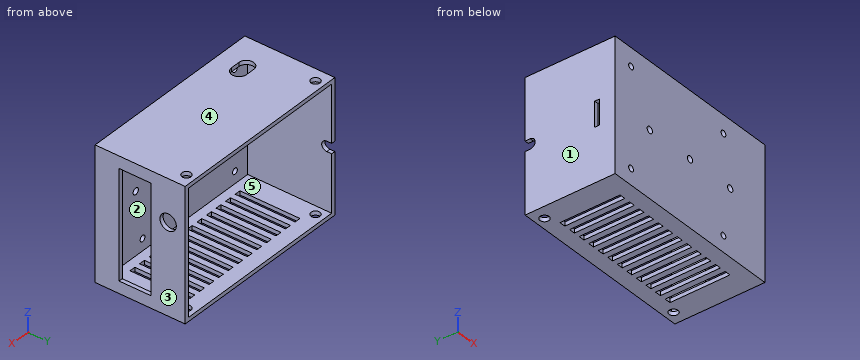
from build123d import *

# Parameters (mm, degrees)
SKETCH1_W           = 90
SKETCH1_H           = 62
BOSS_EXTRUDE1_DEPTH = 3
CUT_EXTRUDE1_REACH  = 56.727
SKETCH2_R           = 1.5
SKETCH3_W           = 94
SKETCH3_H           = 66
SKETCH3_W_2         = 90
SKETCH3_H_2         = 62
BOSS_EXTRUDE2_DEPTH = 45
CUT_EXTRUDE2_REACH  = 109.601
SKETCH4_W           = 12.5
SKETCH4_H           = 2.5
CUT_EXTRUDE3_REACH  = 93.269
CUT_EXTRUDE4_REACH  = 109.601
SKETCH6_W           = 54
SKETCH6_H           = 16
CUT_EXTRUDE5_REACH  = 111.316
SKETCH7_R           = 4.1
SKETCH8_R           = 2.25
CUT_EXTRUDE6_DEPTH  = 93.682252886
CUT_EXTRUDE7_DEPTH  = 72.147733625
CUT_EXTRUDE8_REACH  = 94.682
SKETCH10_W          = 3
SKETCH10_H          = 30
CUT_EXTRUDE9_REACH  = 111.316


with BuildPart() as part:
    # Sketch1 → Boss-Extrude1 (new body)
    with BuildSketch(Plane(origin=(0, 0, 0), x_dir=(1, 0, 0), z_dir=(0, 1, 0))):
        Rectangle(SKETCH1_W, SKETCH1_H)
    extrude(amount=BOSS_EXTRUDE1_DEPTH)

    # Sketch2 → Cut-Extrude1 (cut, up to next)
    with BuildSketch(Plane(origin=(0, 3, 0), x_dir=(1, 0, 0), z_dir=(0, 1, 0)), mode=Mode.PRIVATE) as cut_extrude1_sk1:
        with Locations(Location((-37, -24, 0), (0, 0, 270))):
            Circle(SKETCH2_R)
    cut_extrude1_tool1 = extrude(cut_extrude1_sk1.sketch, amount=-CUT_EXTRUDE1_REACH, mode=Mode.PRIVATE) & part.part
    # Sketch2 → Cut-Extrude1 (cut, up to next)
    with BuildSketch(Plane(origin=(0, 3, 0), x_dir=(1, 0, 0), z_dir=(0, 1, 0)), mode=Mode.PRIVATE) as cut_extrude1_sk2:
        with Locations(Location((21, -24, 0), (0, 0, 270))):
            Circle(SKETCH2_R)
    cut_extrude1_tool2 = extrude(cut_extrude1_sk2.sketch, amount=-CUT_EXTRUDE1_REACH, mode=Mode.PRIVATE) & part.part
    # Sketch2 → Cut-Extrude1 (cut, up to next)
    with BuildSketch(Plane(origin=(0, 3, 0), x_dir=(1, 0, 0), z_dir=(0, 1, 0)), mode=Mode.PRIVATE) as cut_extrude1_sk3:
        with Locations(Location((21, 25, 0), (0, 0, 270))):
            Circle(SKETCH2_R)
    cut_extrude1_tool3 = extrude(cut_extrude1_sk3.sketch, amount=-CUT_EXTRUDE1_REACH, mode=Mode.PRIVATE) & part.part
    # Sketch2 → Cut-Extrude1 (cut, up to next)
    with BuildSketch(Plane(origin=(0, 3, 0), x_dir=(1, 0, 0), z_dir=(0, 1, 0)), mode=Mode.PRIVATE) as cut_extrude1_sk4:
        with Locations(Location((-37, 25, 0), (0, 0, 270))):
            Circle(SKETCH2_R)
    cut_extrude1_tool4 = extrude(cut_extrude1_sk4.sketch, amount=-CUT_EXTRUDE1_REACH, mode=Mode.PRIVATE) & part.part
    add(cut_extrude1_tool1.solids().sort_by_distance((-37, 3, 24))[0], mode=Mode.SUBTRACT)
    add(cut_extrude1_tool2.solids().sort_by_distance((21, 3, 24))[0], mode=Mode.SUBTRACT)
    add(cut_extrude1_tool3.solids().sort_by_distance((21, 3, -25))[0], mode=Mode.SUBTRACT)
    add(cut_extrude1_tool4.solids().sort_by_distance((-37, 3, -25))[0], mode=Mode.SUBTRACT)

    # Sketch3 → Boss-Extrude2 (add)
    with BuildSketch(Plane(origin=(0, 0, 0), x_dir=(1, 0, 0), z_dir=(0, 1, 0))):
        Rectangle(SKETCH3_W, SKETCH3_H)
        Rectangle(SKETCH3_W_2, SKETCH3_H_2, mode=Mode.SUBTRACT)
    extrude(amount=BOSS_EXTRUDE2_DEPTH)

    # Sketch4 → Cut-Extrude2 (cut, up to next)
    with BuildSketch(Plane(origin=(-45, 0, 0), x_dir=(0, 0, -1), z_dir=(1, 0, 0)), mode=Mode.PRIVATE) as cut_extrude2_sk1:
        with Locations((0, 9)):
            Rectangle(SKETCH4_W, SKETCH4_H)
    cut_extrude2_tool1 = extrude(cut_extrude2_sk1.sketch, amount=-CUT_EXTRUDE2_REACH, mode=Mode.PRIVATE) & part.part
    add(cut_extrude2_tool1.solids().sort_by_distance((-45, 9, 0))[0], mode=Mode.SUBTRACT)

    # Sketch5 → Cut-Extrude3 (cut, up to next)
    with BuildSketch(Plane(origin=(0, 0, 31), x_dir=(-1, 0, 0), z_dir=(0, 0, -1)), mode=Mode.PRIVATE) as cut_extrude3_sk1:
        with BuildLine():
            Line((31.55, 9.25), (27.05, 9.25))
            ThreePointArc((27.05, 9.25), (23.3, 13), (27.05, 16.75))
            Line((27.05, 16.75), (31.55, 16.75))
            ThreePointArc((31.55, 16.75), (35.3, 13), (31.55, 9.25))
        make_face()
    cut_extrude3_tool1 = extrude(cut_extrude3_sk1.sketch, amount=-CUT_EXTRUDE3_REACH, mode=Mode.PRIVATE) & part.part
    add(cut_extrude3_tool1.solids().sort_by_distance((-29.3, 13, 31))[0], mode=Mode.SUBTRACT)

    # Sketch6 → Cut-Extrude4 (cut, up to next)
    with BuildSketch(Plane.ZY.offset(-45), mode=Mode.PRIVATE) as cut_extrude4_sk1:
        with Locations((0, 20)):
            Rectangle(SKETCH6_W, SKETCH6_H)
    cut_extrude4_tool1 = extrude(cut_extrude4_sk1.sketch, amount=-CUT_EXTRUDE4_REACH, mode=Mode.PRIVATE) & part.part
    add(cut_extrude4_tool1.solids().sort_by_distance((45, 20, 0))[0], mode=Mode.SUBTRACT)

    # Sketch7 → Cut-Extrude5 (cut, up to next)
    with BuildSketch(Plane(origin=(47, 0, 0), x_dir=(0, 0, -1), z_dir=(1, 0, 0)), mode=Mode.PRIVATE) as cut_extrude5_sk1:
        with Locations((-12, 36.5)):
            Circle(SKETCH7_R)
    cut_extrude5_tool1 = extrude(cut_extrude5_sk1.sketch, amount=-CUT_EXTRUDE5_REACH, mode=Mode.PRIVATE) & part.part
    add(cut_extrude5_tool1.solids().sort_by_distance((47, 36.5, 12))[0], mode=Mode.SUBTRACT)

    # Sketch8 → Cut-Extrude6 (cut, through all)
    with BuildSketch(Plane.XY.offset(33)):
        with Locations((-40.5, 40.5)):
            Circle(SKETCH8_R)
        with Locations(Location((40.5, 40.5, 0), (0, 0, 180))):
            Circle(SKETCH8_R)
    extrude(amount=-CUT_EXTRUDE6_DEPTH, mode=Mode.SUBTRACT)

    # Sketch9 → Cut-Extrude7 (cut, through all)
    with BuildSketch(Plane(origin=(0, 3, 0), x_dir=(1, 0, 0), z_dir=(0, 1, 0))):
        with BuildLine():
            ThreePointArc((-23.6, 0), (-25.25, 1.65), (-26.9, 0))
            Line((-26.9, 0), (-23.6, 0))
        make_face()
        with BuildLine():
            Line((-23.6, 0), (-26.9, 0))
            ThreePointArc((-26.9, 0), (-25.25, -1.65), (-23.6, 0))
        make_face()
        with BuildLine():
            ThreePointArc((1.65, 0), (0, 1.65), (-1.65, 0))
            Line((-1.65, 0), (1.65, 0))
        make_face()
        with BuildLine():
            Line((1.65, 0), (-1.65, 0))
            ThreePointArc((-1.65, 0), (0, -1.65), (1.65, 0))
        make_face()
        with BuildLine():
            ThreePointArc((26.9, 0), (25.25, 1.65), (23.6, 0))
            Line((23.6, 0), (26.9, 0))
        make_face()
        with BuildLine():
            Line((26.9, 0), (23.6, 0))
            ThreePointArc((23.6, 0), (25.25, -1.65), (26.9, 0))
        make_face()
    extrude(amount=-CUT_EXTRUDE7_DEPTH, mode=Mode.SUBTRACT)

    # Sketch10 → Cut-Extrude8 (cut, up to next)
    with BuildSketch(Plane(origin=(0, 0, -33), x_dir=(-1, 0, 0), z_dir=(0, 0, -1)), mode=Mode.PRIVATE) as cut_extrude8_sk1:
        with Locations((9, 22.5)):
            Rectangle(SKETCH10_W, SKETCH10_H)
    cut_extrude8_tool1 = extrude(cut_extrude8_sk1.sketch, amount=-CUT_EXTRUDE8_REACH, mode=Mode.PRIVATE) & part.part
    # Sketch10 → Cut-Extrude8 (cut, up to next)
    with BuildSketch(Plane(origin=(0, 0, -33), x_dir=(-1, 0, 0), z_dir=(0, 0, -1)), mode=Mode.PRIVATE) as cut_extrude8_sk2:
        with Locations((3, 22.5)):
            Rectangle(SKETCH10_W, SKETCH10_H)
    cut_extrude8_tool2 = extrude(cut_extrude8_sk2.sketch, amount=-CUT_EXTRUDE8_REACH, mode=Mode.PRIVATE) & part.part
    # Sketch10 → Cut-Extrude8 (cut, up to next)
    with BuildSketch(Plane(origin=(0, 0, -33), x_dir=(-1, 0, 0), z_dir=(0, 0, -1)), mode=Mode.PRIVATE) as cut_extrude8_sk3:
        with Locations((15, 22.5)):
            Rectangle(SKETCH10_W, SKETCH10_H)
    cut_extrude8_tool3 = extrude(cut_extrude8_sk3.sketch, amount=-CUT_EXTRUDE8_REACH, mode=Mode.PRIVATE) & part.part
    # Sketch10 → Cut-Extrude8 (cut, up to next)
    with BuildSketch(Plane(origin=(0, 0, -33), x_dir=(-1, 0, 0), z_dir=(0, 0, -1)), mode=Mode.PRIVATE) as cut_extrude8_sk4:
        with Locations((21, 22.5)):
            Rectangle(SKETCH10_W, SKETCH10_H)
    cut_extrude8_tool4 = extrude(cut_extrude8_sk4.sketch, amount=-CUT_EXTRUDE8_REACH, mode=Mode.PRIVATE) & part.part
    # Sketch10 → Cut-Extrude8 (cut, up to next)
    with BuildSketch(Plane(origin=(0, 0, -33), x_dir=(-1, 0, 0), z_dir=(0, 0, -1)), mode=Mode.PRIVATE) as cut_extrude8_sk5:
        with Locations((27, 22.5)):
            Rectangle(SKETCH10_W, SKETCH10_H)
    cut_extrude8_tool5 = extrude(cut_extrude8_sk5.sketch, amount=-CUT_EXTRUDE8_REACH, mode=Mode.PRIVATE) & part.part
    # Sketch10 → Cut-Extrude8 (cut, up to next)
    with BuildSketch(Plane(origin=(0, 0, -33), x_dir=(-1, 0, 0), z_dir=(0, 0, -1)), mode=Mode.PRIVATE) as cut_extrude8_sk6:
        with Locations((33, 22.5)):
            Rectangle(SKETCH10_W, SKETCH10_H)
    cut_extrude8_tool6 = extrude(cut_extrude8_sk6.sketch, amount=-CUT_EXTRUDE8_REACH, mode=Mode.PRIVATE) & part.part
    # Sketch10 → Cut-Extrude8 (cut, up to next)
    with BuildSketch(Plane(origin=(0, 0, -33), x_dir=(-1, 0, 0), z_dir=(0, 0, -1)), mode=Mode.PRIVATE) as cut_extrude8_sk7:
        with Locations((-3, 22.5)):
            Rectangle(SKETCH10_W, SKETCH10_H)
    cut_extrude8_tool7 = extrude(cut_extrude8_sk7.sketch, amount=-CUT_EXTRUDE8_REACH, mode=Mode.PRIVATE) & part.part
    # Sketch10 → Cut-Extrude8 (cut, up to next)
    with BuildSketch(Plane(origin=(0, 0, -33), x_dir=(-1, 0, 0), z_dir=(0, 0, -1)), mode=Mode.PRIVATE) as cut_extrude8_sk8:
        with Locations((-9, 22.5)):
            Rectangle(SKETCH10_W, SKETCH10_H)
    cut_extrude8_tool8 = extrude(cut_extrude8_sk8.sketch, amount=-CUT_EXTRUDE8_REACH, mode=Mode.PRIVATE) & part.part
    # Sketch10 → Cut-Extrude8 (cut, up to next)
    with BuildSketch(Plane(origin=(0, 0, -33), x_dir=(-1, 0, 0), z_dir=(0, 0, -1)), mode=Mode.PRIVATE) as cut_extrude8_sk9:
        with Locations((-15, 22.5)):
            Rectangle(SKETCH10_W, SKETCH10_H)
    cut_extrude8_tool9 = extrude(cut_extrude8_sk9.sketch, amount=-CUT_EXTRUDE8_REACH, mode=Mode.PRIVATE) & part.part
    # Sketch10 → Cut-Extrude8 (cut, up to next)
    with BuildSketch(Plane(origin=(0, 0, -33), x_dir=(-1, 0, 0), z_dir=(0, 0, -1)), mode=Mode.PRIVATE) as cut_extrude8_sk10:
        with Locations((-21, 22.5)):
            Rectangle(SKETCH10_W, SKETCH10_H)
    cut_extrude8_tool10 = extrude(cut_extrude8_sk10.sketch, amount=-CUT_EXTRUDE8_REACH, mode=Mode.PRIVATE) & part.part
    # Sketch10 → Cut-Extrude8 (cut, up to next)
    with BuildSketch(Plane(origin=(0, 0, -33), x_dir=(-1, 0, 0), z_dir=(0, 0, -1)), mode=Mode.PRIVATE) as cut_extrude8_sk11:
        with Locations((-27, 22.5)):
            Rectangle(SKETCH10_W, SKETCH10_H)
    cut_extrude8_tool11 = extrude(cut_extrude8_sk11.sketch, amount=-CUT_EXTRUDE8_REACH, mode=Mode.PRIVATE) & part.part
    # Sketch10 → Cut-Extrude8 (cut, up to next)
    with BuildSketch(Plane(origin=(0, 0, -33), x_dir=(-1, 0, 0), z_dir=(0, 0, -1)), mode=Mode.PRIVATE) as cut_extrude8_sk12:
        with Locations((-33, 22.5)):
            Rectangle(SKETCH10_W, SKETCH10_H)
    cut_extrude8_tool12 = extrude(cut_extrude8_sk12.sketch, amount=-CUT_EXTRUDE8_REACH, mode=Mode.PRIVATE) & part.part
    add(cut_extrude8_tool1.solids().sort_by_distance((-9, 22.5, -33))[0], mode=Mode.SUBTRACT)
    add(cut_extrude8_tool2.solids().sort_by_distance((-3, 22.5, -33))[0], mode=Mode.SUBTRACT)
    add(cut_extrude8_tool3.solids().sort_by_distance((-15, 22.5, -33))[0], mode=Mode.SUBTRACT)
    add(cut_extrude8_tool4.solids().sort_by_distance((-21, 22.5, -33))[0], mode=Mode.SUBTRACT)
    add(cut_extrude8_tool5.solids().sort_by_distance((-27, 22.5, -33))[0], mode=Mode.SUBTRACT)
    add(cut_extrude8_tool6.solids().sort_by_distance((-33, 22.5, -33))[0], mode=Mode.SUBTRACT)
    add(cut_extrude8_tool7.solids().sort_by_distance((3, 22.5, -33))[0], mode=Mode.SUBTRACT)
    add(cut_extrude8_tool8.solids().sort_by_distance((9, 22.5, -33))[0], mode=Mode.SUBTRACT)
    add(cut_extrude8_tool9.solids().sort_by_distance((15, 22.5, -33))[0], mode=Mode.SUBTRACT)
    add(cut_extrude8_tool10.solids().sort_by_distance((21, 22.5, -33))[0], mode=Mode.SUBTRACT)
    add(cut_extrude8_tool11.solids().sort_by_distance((27, 22.5, -33))[0], mode=Mode.SUBTRACT)
    add(cut_extrude8_tool12.solids().sort_by_distance((33, 22.5, -33))[0], mode=Mode.SUBTRACT)

    # Sketch11 → Cut-Extrude9 (cut, up to next)
    with BuildSketch(Plane.ZY.offset(47), mode=Mode.PRIVATE) as cut_extrude9_sk1:
        with BuildLine():
            Line((2.5, 47.5), (2.5, 42.5))
            ThreePointArc((2.5, 42.5), (0, 40), (-2.5, 42.5))
            Line((-2.5, 42.5), (-2.5, 47.5))
            ThreePointArc((-2.5, 47.5), (0, 50), (2.5, 47.5))
        make_face()
    cut_extrude9_tool1 = extrude(cut_extrude9_sk1.sketch, amount=-CUT_EXTRUDE9_REACH, mode=Mode.PRIVATE) & part.part
    add(cut_extrude9_tool1.solids().sort_by_distance((-47, 45, 0))[0], mode=Mode.SUBTRACT)


solid = part.part
Source: CAD feature listing. Evaluate the final solid. Frame: model axes, mm. Face numbers are marked on the shaded views. A direction names the side the tool comes from. Round coordinates to 2 decimals unless told otherwise and drop trailing zeros. Loops run counter-clockwise (first coordinate to the right, second up) from the corner with the lowest first, then second, coordinate; pieces in that order, holes last. Notation, with made-up numbers: (-24.75, -24.5) - (-20.75, -24.5) arc R21 cw to (-20.75, 5.5) - close; hole circle Ø2 at (31, 29). An arc over 180 degrees is marked (long way). Write item = value, one per line. Start each with the question number.
Item 1: Section query B-B on z = -25. Output: boundary loops of the cut face in (x, y), plus the area to 3 significant figures.
Item 2: Section query C-C on y = 13. Count the separate pieces of the cut face and the enclosed holes in it, plus the area to 3 significant figures.
Item 3: Reachability of the marked faces 1 and 2 from +Z, -Z, +X, -X, +Y, -Y: full face, straight path, thin tool, end or side. Return the list, or none.
Item 4: Section query D-D on z = 29. Output: boundary loops of the cut face in (x, y).
Item 5: Mould query, pull axis Z, two halves, no side actions, for the marked faces 3, 4 and 5. Classes: released by +Z, released by -Z, zero draft, split by the parting line, or undercut.
Item 6: Material intervals for line 1 (Z direction, x = 5.5, y = 26.5); line 2 (X direction, y = 41, z = -6); line 3 (Y direction, x = 2, z = -28), sorted ascending.
Item 7: First-contact query: pin 1 Ø3 at (y, z) = (21, -0.5) entering from +X; pin 2 Ø6 at (x, z) = (16, -0.5) entering from +Y; pin 3 Ø1 at (x, z) = (-46, -0.5) entering from +Y; pin 4 Ø0.6 at (x, z) = (8.5, -32) entering from -Y. Flat tips, straight axial feed; report the tip coordinate or a pass-through.
Item 8: Section query A-A on x = -40.5. Output: boundary loops of the cut face in (y, z), plus the area to 3 significant figures.
Results list:
q1.outline = (-47, 0) - (-38.5, 0) - (-38.5, 3) - (-45, 3) - (-45, 45) - (-47, 45) - close; (-35.5, 0) - (19.5, 0) - (19.5, 3) - (-35.5, 3) - close; (22.5, 0) - (47, 0) - (47, 12) - (45, 12) - (45, 3) - (22.5, 3) - close; (45, 28) - (47, 28) - (47, 45) - (45, 45) - close
q1.area = 400 mm²
q2.separate_pieces = 14
q2.enclosed_holes = 0
q2.area = 420 mm²
q3.face_1 = +Z, -Z, -X, +Y, -Y
q3.face_2 = +Y
q4.outline = (-47, 0) - (47, 0) - (47, 45) - (45, 45) - (45, 3) - (-45, 3) - (-45, 45) - (-47, 45) - close
q5.face_3 = zero draft
q5.face_4 = released by +Z
q5.face_5 = undercut
q6.line_1 = -33 to -31, 31 to 33
q6.line_2 = -47 to -45, 45 to 47
q6.line_3 = 0 to 3
q7.pin_1 = -45
q7.pin_2 = 3
q7.pin_3 = 40.21
q7.pin_4 = 0
q8.outline = (0, -33) - (38.25, -33) - (38.25, -31) - (3, -31) - (3, 31) - (38.25, 31) - (38.25, 33) - (0, 33) - close; (42.75, -33) - (45, -33) - (45, -31) - (42.75, -31) - close; (42.75, 31) - (45, 31) - (45, 33) - (42.75, 33) - close
q8.area = 348 mm²
